Job drawing, mm, ordinate dimensions from the low corner. One solid piece. A direction names the side the tool comes from. Round coordinates to 2 decimals unless told otherwise and drop trailing zeros. Loops run counter-clockwise (first coordinate to the right, second up) from the corner with the lowest first, then second, coordinate; pieces in that order, holes last.
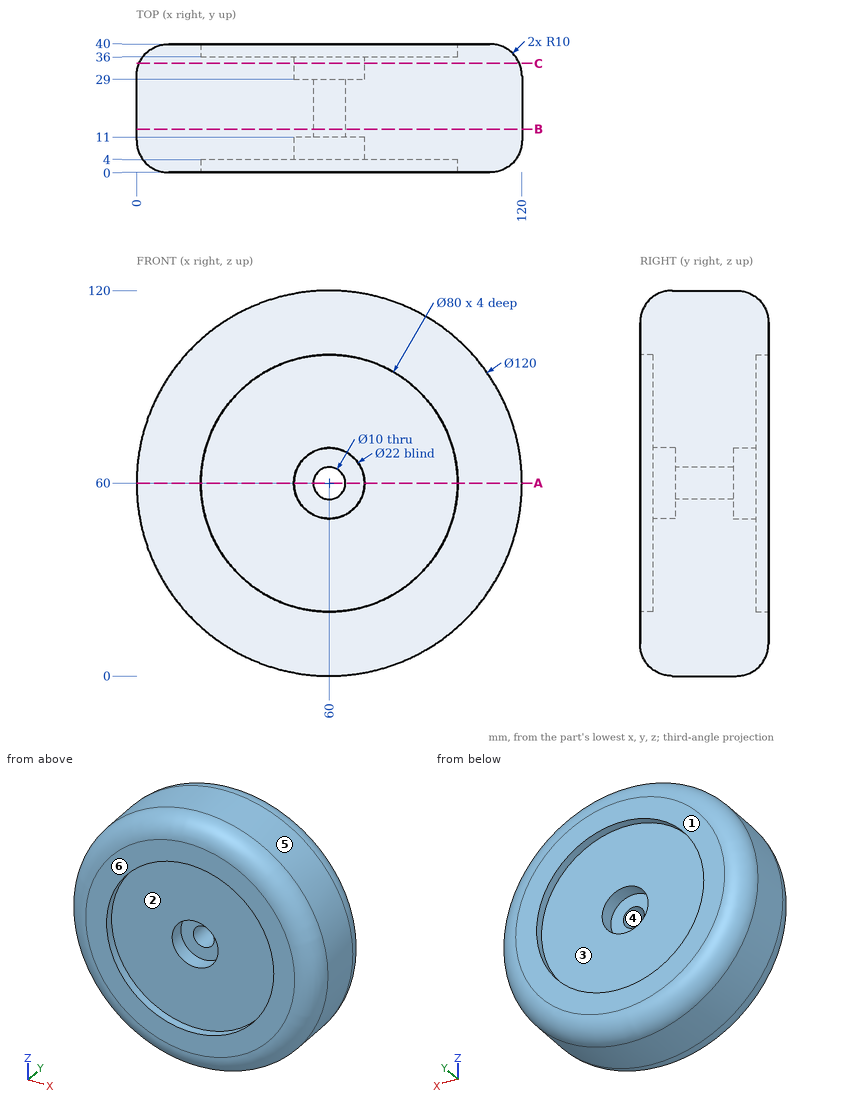
1) Slice it at C-C, the plane y = 34. Give the cut face in (x, z), then the cut area to 3 significant figures.
Values:
outline: circle Ø118.33 at (60, 60); hole circle Ø22 at (60, 60)
area: 10,600 mm2
2) Mould opens along X. For the marked faces 4, 5 and 6 say: released by +X, released by -X, zero draft, split by the parting line, or undercut.
Values:
face 4: undercut
face 5: split by the parting line
face 6: zero draft
3) Drop flat-ended pins along their axis: pin 1 Ø8 at (y, z) = (30.5, 21) entering from +X; pin 2 Ø9 at (x, z) = (60, 60) entering from -Y; pin 3 Ø2 at (x, y) = (70.5, 12) entering from -Z; pin 4 Ø24 at (x, z) = (73.5, 52.5) entering from -Y. Give the stop position or say it passes through.
Values:
pin 1: stops at x = 108.72
pin 2: passes through
pin 3: stops at z = 0.76
pin 4: stops at y = 4
4) Slice it at B-B, the plane y = 13.5. Give the cut face in (x, z), then the cut area to 3 significant figures.
Values:
outline: circle Ø120 at (60, 60); hole circle Ø10 at (60, 60)
area: 11,200 mm2
5) Slice it at A-A, the plane z = 60. Give the cut face in (x, y), then the cut area to 3 significant figures.
Values:
outline: (0, 10) arc R10 ccw to (10, 0) - (20, 0) - (20, 4) - (49, 4) - (49, 11) - (55, 11) - (55, 29) - (49, 29) - (49, 36) - (20, 36) - (20, 40) - (10, 40) arc R10 ccw to (0, 30) - close; (65, 11) - (71, 11) - (71, 4) - (100, 4) - (100, 0) - (110, 0) arc R10 ccw to (120, 10) - (120, 30) arc R10 ccw to (110, 40) - (100, 40) - (100, 36) - (71, 36) - (71, 29) - (65, 29) - close
area: 3,590 mm2
6) Tool access for the marked faces 1, 2 and 3: list every direction of +Z, -Z, +X, -X, +Y, -Y with a clear straight run to the whole face (end or side of a thin tool).
Values:
face 1: +Z, -Z, +X, -X, +Y
face 2: -Y
face 3: +Y
7) Wall check: line 1 along Z through (x, y) = (60, 16); line 2 along Y through (x, z) = (62.5, 85.5); line 3 along X through (y, z) = (27, 58). Give the ranges that are in metal, low to high.
Values:
line 1: z = 0 to 55, 65 to 120
line 2: y = 4 to 36
line 3: x = 0.03 to 55.42, 64.58 to 119.97
